Can you work these out from the model? Positions are in its coordinate system, mm. Round coordinates to 2 decimals unless told otherwise and drop trailing zeros. Order: outer loops, then holes, each group sorted by start corner. A loop starts at its lowest first (then second) coordinate and runs counter-clockwise, first axis right, second up. Notation, with made-up numbers: M 50.25,15.25 L 81.25,15.25 A32 cw 81.25,54.25 Z; hole C -29,-33 d6. An arc over 180 degrees is marked long. Answer as a JSON object with one key per item and string values. Group by question number.
from build123d import *

# Parameters (mm, degrees)
F0_W     = 76.2
F0_H     = 27.3757269502
F0_H_2   = 48.8242730498
F0_R     = 9.4325201181
F0_R_2   = 8.8008195624
F1_DEPTH = 25.4


with BuildPart() as f1:
    # F0 (on Top) → F1 (new body)
    with BuildSketch(Plane.XY):
        with Locations((-8.3431932092, 28.7107112765)):
            Rectangle(F0_W, F0_H)
        with Locations((-8.3431932092, -9.3892887235)):
            Rectangle(F0_W, F0_H_2)
        with Locations((-29.7568067908, -5.7780258358)):
            Circle(F0_R, mode=Mode.SUBTRACT)
        with Locations((13.5783478618, -5.7780258358)):
            Circle(F0_R_2, mode=Mode.SUBTRACT)
    extrude(amount=F1_DEPTH)


solid = f1.part
Item 1: Suppose I cut it at C-C, the plane x = -35. Write out the boundary of the cut face in (y, z), and give its area (3 significant figures).
Item 2: Suppose I cut it at A-A, the plane x = -27. Write out the boundary of the cut face in (y, z).
Item 3: I need wall thicknesses on line 1 (X direction, y = -5, z = 7); line 2 (X direction, y = -4, z = 15); line 3 (Y direction, x = -30, z = 4.75). Which ranges of each line are inside material? Lowest first, please.
Item 4: Suppose I cut it at B-B, the plane z = 17. Write out the boundary of the cut face in (x, y), and give its area (3 significant figures).
Computed:
{
 "1": {"outline": "M -33.8,0 L -13.62,0 L -13.62,25.4 L -33.8,25.4 Z; M 2.06,0 L 42.4,0 L 42.4,25.4 L 2.06,25.4 Z", "area": "1,540 mm^2"},
 "2": {"outline": "M -33.8,0 L -14.8,0 L -14.8,25.4 L -33.8,25.4 Z; M 3.24,0 L 42.4,0 L 42.4,25.4 L 3.24,25.4 Z"},
 "3": {"line 1": "x = -46.44 to -39.16, -20.36 to 4.81, 22.34 to 29.76", "line 2": "x = -46.44 to -39.02, -20.49 to 4.96, 22.2 to 29.76", "line 3": "y = -33.8 to -15.21, 3.65 to 42.4"},
 "4": {"outline": "M -46.44,-33.8 L 29.76,-33.8 L 29.76,42.4 L -46.44,42.4 Z; hole C -29.76,-5.78 d18.87; hole C 13.58,-5.78 d17.6", "area": "5,280 mm^2"}
}
